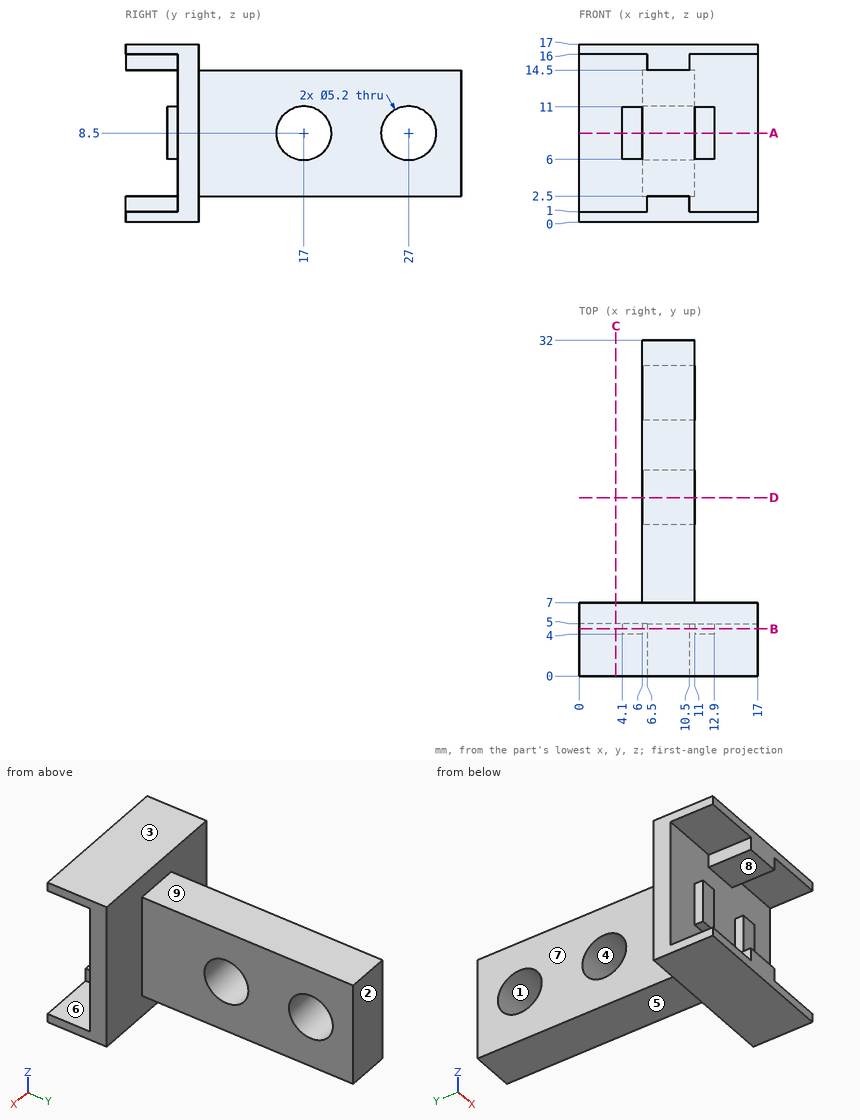
Check sheet for the drawn part. Datum: minimum x, y, z corner. Units: mm. A direction names the side the tool comes from. Give positions to 0.01 mm unless a question says otherwise; leave off trailing zeros. Write each loop counter-clockwise with the first axis right and the second up, starting at its lowest first coordinate (ties: lowest second). Pieces come first, ordered by that corner, then holes. Notation, with made-up numbers: (-31.5, 44) -> (7.5, 44) arc R30 ccw to (7.5, 74) -> close; hole circle Ø3 at (-17, 39.25). An arc over 180 degrees is marked (long way). Use one line per item in the form item = value. Start each with the question number.
1. Section check A-A (z = 8.5). Record the cut outline in (x, y).
2. Go/stop test with flat-tipped pins: P1, Ø9.5, axis at y = 23, z = 5.5, coming from the -X side; P2, Ø2, axis at y = 10.5, z = 6.5, coming from the +X side; P3, Ø1.5, axis at x = 13, z = 5.5, coming from the +Y side; P4, Ø4.5, axis at y = 17, z = 8.5, coming from the -X side. Record where each tip stops, or that it passes through.
3. Section check D-D (y = 17). Record the cut outline in (x, z).
4. Section check B-B (y = 4.5). Record the cut outline in (x, z), and give its area (3 significant figures).
5. Mould release check, pull along Y, two halves, no side actions. Record for the marked faces 1, 2, 3 and 4: pulls with the +Y half, pulls with the -Y half, needs draft (parallel to the pull), parting line crosses it, or undercut.
6. Section check C-C (x = 3.5). Record the cut outline in (y, z), and give its area (3 significant figures).
7. Access from +Z, -Z, +X, -X, +Y, -Y to the whole of each face (thin tool, end or side, straight path). Record for the marked faces 5, 6, 7, 8 and 9.
8. Thickness scan on line 1 along Y through (x, z) = (9.2, 8.5); line 2 along Y through (x, z) = (16, 7); line 3 along X through (y, z) = (8, 3.5). Record the ranges inside material, lowest first. Write a range as from..to.
Conclusion:
q1.outline = (0, 5) -> (4.1, 5) -> (4.1, 4) -> (6, 4) -> (6, 5) -> (11, 5) -> (11, 4) -> (12.9, 4) -> (12.9, 5) -> (17, 5) -> (17, 7) -> (11, 7) -> (11, 14.4) -> (6, 14.4) -> (6, 7) -> (0, 7) -> close; (6, 19.6) -> (11, 19.6) -> (11, 24.4) -> (6, 24.4) -> close; (6, 29.6) -> (11, 29.6) -> (11, 32) -> (6, 32) -> close
q2.P1 = 6
q2.P2 = 11
q2.P3 = 7
q2.P4 = through
q3.outline = (6, 2.5) -> (11, 2.5) -> (11, 5.9) -> (6, 5.9) -> close; (6, 11.1) -> (11, 11.1) -> (11, 14.5) -> (6, 14.5) -> close
q4.outline = (0, 0) -> (17, 0) -> (17, 1) -> (10.5, 1) -> (10.5, 2.5) -> (6.5, 2.5) -> (6.5, 1) -> (0, 1) -> close; (0, 16) -> (6.5, 16) -> (6.5, 14.5) -> (10.5, 14.5) -> (10.5, 16) -> (17, 16) -> (17, 17) -> (0, 17) -> close; (4.1, 6) -> (6, 6) -> (6, 11) -> (4.1, 11) -> close; (11, 6) -> (12.9, 6) -> (12.9, 11) -> (11, 11) -> close
q4.area = 65.0 mm²
q5.face_1 = undercut
q5.face_2 = pulls with the +Y half
q5.face_3 = needs draft
q5.face_4 = undercut
q6.outline = (0, 0) -> (7, 0) -> (7, 17) -> (0, 17) -> (0, 16) -> (5, 16) -> (5, 1) -> (0, 1) -> close
q6.area = 44.0 mm²
q7.face_5 = -Z, +X, -X, +Y
q7.face_6 = +X, -Y
q7.face_7 = +Z, -Z, -X, +Y
q7.face_8 = +X, -X, -Y
q7.face_9 = +Z, +X, -X, +Y
q8.line_1 = 5..14.4, 19.6..24.4, 29.6..32
q8.line_2 = 5..7
q8.line_3 = 6..11
